Read the model definition and answer for the solid it produces. Units are mm, in the model's axes. A direction names the side the tool comes from. Give positions to 0.01 mm unless a question says otherwise; leave off trailing zeros. Order: outer loops, then holes, each group sorted by start corner. A loop starts at its lowest first (then second) coordinate and runs counter-clockwise, first axis right, second up.
Item 1: Find the intervals of material crossed by line 1 along Y through (x, z) = (70, -89); line 2 along Y through (x, z) = (62, -104); line 3 along X through (y, z) = (-12, -112.5), in increasing order.
Item 2: Given pin 1 Ø6 at (y, z) = (1.5, -111.5) entering from +X; pin 2 Ø1.5 at (x, z) = (54, -89) entering from -Y; pin 3 Ø6 at (x, z) = (94.5, -28) entering from +Y, each flat-ended and moving along its own axis, determine where each tip first touches the part or whether it passes through.
Item 3: Which of the six approach directions +Z, -Z, +X, -X, +Y, -Y give full straight-line access (tool end or side, diameter ignored) to faces 1 (the face through (60, -26, -125)), 2 (the face through (37.67, -13.41, -129.56))?
Item 4: The mould has two halves that part along X. Classify faces 3 (the face through (42.363, -2.758, -129.93)), 4 (the face through (45.024, -1.099, -61.146)), 5 (the face through (89.98, 0.88, -68.43)), 6 (the face through (70.1, -21.2, 0)): +X half, -X half, draft (parallel to the pull), parting line (faces both ways), or undercut.
Item 5: A cutting plane is placed at B-B (z = -56.5). Write down the section's boundary in (x, y), plus the area to 3 significant figures.
Item 6: A cutting plane is placed at A-A (x = 70). Write down the section's boundary in (y, z).
from build123d import *

# Parameters (mm, degrees)
SKETCH_1_R                = 35
EXTRUDE_1_DEPTH           = 5
SKETCH_2_R                = 25
EXTRUDE_2_DEPTH           = 135
SKETCH_4_R                = 35
CUT_EXTRUDE_2_DEPTH       = 5
SKETCH_9_R                = 35
EXTRUDE_3_DEPTH           = 10
CHAMFER_1_SIZE            = 1
HOLE_WIZARD_M6_1_D        = 5
HOLE_WIZARD_M6_1_DEPTH    = 25
HOLE_WIZARD_M6_1_TIP      = 1.502151548
HOLE_WIZARD_6_0_6_1_D     = 6
HOLE_WIZARD_6_0_6_1_DEPTH = 20
HOLE_WIZARD_6_0_6_1_TIP   = 1.802581857
CHAMFER_2_SIZE            = 0.5
SKETCH_10_R               = 20
CUT_EXTRUDE_3_DEPTH       = 175.570902501
FILLET_1_R                = 2
CHAMFER_3_SIZE            = 1


with BuildPart() as part:
    # 草图1 → 凸台-拉伸1 (new body)
    with BuildSketch(Plane.XY):
        with Locations((70, 0)):
            Circle(SKETCH_1_R)
    extrude(amount=EXTRUDE_1_DEPTH)

    # 草图2 → 凸台-拉伸2 (add)
    with BuildSketch(Plane(origin=(0, 0, 0), x_dir=(-1, 0, 0), z_dir=(0, 0, -1))):
        with Locations(Location((-70, 0, 0), (0, 0, 180))):
            Circle(SKETCH_2_R)
    extrude(amount=EXTRUDE_2_DEPTH)

    # 草图4 → 切除-拉伸2 (cut)
    with BuildSketch(Plane(origin=(0, 0, 0), x_dir=(-1, 0, 0), z_dir=(0, 0, -1))):
        with Locations((-70, 0)):
            Circle(SKETCH_4_R)
    extrude(amount=-CUT_EXTRUDE_2_DEPTH, mode=Mode.SUBTRACT)

    # 草图9 → 凸台-拉伸3 (add)
    with BuildSketch(Plane(origin=(0, 0, -135), x_dir=(-1, 0, 0), z_dir=(0, 0, -1))):
        with Locations((-70, 0)):
            Circle(SKETCH_9_R)
    extrude(amount=-EXTRUDE_3_DEPTH)

    # 倒角1
    chamfer_1_edges = [part.edges().sort_by_distance(p)[0] for p in [
        (105, 0, -135),
        (45, 0, 0),
    ]]
    chamfer(chamfer_1_edges, length=CHAMFER_1_SIZE)

    # M6 螺纹孔1
    with Locations(Plane(origin=(0, 0, -135), x_dir=(-1, 0, 0), z_dir=(0, 0, -1))):
        with Locations((-62.458195458, -29.036549111), (-95.284853471, -16.145469487), (-59.034192698, 27.924023174), (-40.054054986, -1.800104779)):
            Hole(HOLE_WIZARD_M6_1_D / 2, depth=HOLE_WIZARD_M6_1_DEPTH)
            with Locations((0, 0, -(HOLE_WIZARD_M6_1_DEPTH + HOLE_WIZARD_M6_1_TIP / 2))):  # 118° drill point
                Cone(0, HOLE_WIZARD_M6_1_D / 2, HOLE_WIZARD_M6_1_TIP, mode=Mode.SUBTRACT)

    # Ø6.0 (6) 直径孔1
    with Locations(Plane(origin=(0, 0, -135), x_dir=(-1, 0, 0), z_dir=(0, 0, -1))):
        with Locations((-93.168703387, 19.058100203)):
            Hole(HOLE_WIZARD_6_0_6_1_D / 2, depth=HOLE_WIZARD_6_0_6_1_DEPTH)
            with Locations((0, 0, -(HOLE_WIZARD_6_0_6_1_DEPTH + HOLE_WIZARD_6_0_6_1_TIP / 2))):  # 118° drill point
                Cone(0, HOLE_WIZARD_6_0_6_1_D / 2, HOLE_WIZARD_6_0_6_1_TIP, mode=Mode.SUBTRACT)

    # 倒角2
    chamfer_2_edges = [part.edges().sort_by_distance(p)[0] for p in [
        (90.168703387, 19.058100203, -135),
    ]]
    chamfer(chamfer_2_edges, length=CHAMFER_2_SIZE)

    # 草图10 → 切除-拉伸3 (cut, through all)
    with BuildSketch(Plane(origin=(0, 0, -135), x_dir=(-1, 0, 0), z_dir=(0, 0, -1))):
        with Locations((-70, 0)):
            Circle(SKETCH_10_R)
    extrude(amount=-CUT_EXTRUDE_3_DEPTH, mode=Mode.SUBTRACT)

    # 圆角1
    fillet_1_edges = [part.edges().sort_by_distance(p)[0] for p in [
        (45, 0, -125),
    ]]
    fillet(fillet_1_edges, radius=FILLET_1_R - 0.0001)  # a hair under: the kernel refuses the full size

    # 倒角3
    chamfer_3_edges = [part.edges().sort_by_distance(p)[0] for p in [
        (90, 0, 0),
        (90, 0, -135),
    ]]
    chamfer(chamfer_3_edges, length=CHAMFER_3_SIZE)


solid = part.part
Response values:
1. line 1: y = -25 to -20, 20 to 25
1. line 2: y = -23.69 to -18.33, 18.33 to 23.69
1. line 3: x = 48.07 to 54, 86 to 91.93
2. pin 1: stops at x = 95
2. pin 2: stops at y = -19.81
2. pin 3: stops at y = 12.76
3. face 1: +Z
3. face 2: +Z, -Z
4. face 3: undercut
4. face 4: parting line
4. face 5: undercut
4. face 6: draft
5. outline: circle Ø50 at (70, 0); hole circle Ø40 at (70, 0)
5. area: 707 mm2
6. outline: (-35, -134) - (-34, -135) - (-21, -135) - (-20, -134) - (-20, -1) - (-21, 0) - (-24, 0) - (-25, -1) - (-25, -123) arc R2 cw to (-27, -125) - (-35, -125) - close; (20, -134) - (21, -135) - (34, -135) - (35, -134) - (35, -125) - (27, -125) arc R2 cw to (25, -123) - (25, -1) - (24, 0) - (21, 0) - (20, -1) - close
